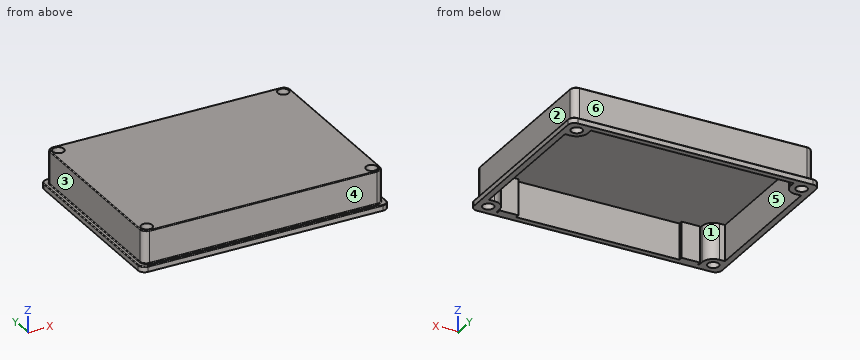
Autodesk Inventor part; units mm, degrees
ref_plane "YZ Plane" through (0, 0, 0) normal (1, 0, 0) x (0, 1, 0)
ref_plane "XZ Plane" through (0, 0, 0) normal (0, 1, 0) x (-1, 0, 0)
ref_plane "XY Plane" through (0, 0, 0) normal (0, 0, 1) x (1, 0, 0)
sketch "Sketch1" plane through (0, 0, 0) normal (0, 0, 1) x (1, 0, 0)
  line L0 (-150, 110) -> (150, 110)
  line L1 (150, 110) -> (150, -110)
  line L2 (150, -110) -> (-150, -110)
  line L3 (-150, -110) -> (-150, 110)
  line L4 (-150, 110) -> (150, -110) construction
  line L5 (150, 110) -> (-150, -110) construction
  point P0 (0, 0)
  dimension "d0" = 300
  dimension "d1" = 220
extrude "Extrusion1" add sketch "Sketch1" along normal blind 48
sketch "Sketch2" plane through (0, 0, 0) normal (0, 0, 1) x (1, 0, 0)
  line L0 (-155, -115) -> (155, -115)
  line L1 (155, -115) -> (155, 115)
  line L2 (155, 115) -> (-155, 115)
  line L3 (-155, 115) -> (-155, -115)
  line L4 (-155, -115) -> (155, 115) construction
  line L5 (155, -115) -> (-155, 115) construction
  point P0 (0, 0)
  dimension "d4" = 310
  dimension "d5" = 230
extrude "Extrusion2" add sketch "Sketch2" along normal blind 7
fillet "Fillet1" radius 8 8 edges at (-150, -110, 27.5) (-155, -115, 3.5) (155, -115, 3.5) (150, -110, 27.5) (155, 115, 3.5) (150, 110, 27.5) (-155, 115, 3.5) (-150, 110, 27.5)
fillet "Fillet2" radius 1 24 edges at (152.6569, -112.6569, 7) (155, 0, 7) (152.6569, 112.6569, 7) (0, 115, 7) (-152.6569, 112.6569, 7) (-155, 0, 7) (-152.6569, -112.6569, 7) (0, -115, 7) (147.6569, -107.6569, 7) (150, 0, 7) (147.6569, 107.6569, 7) (0, 110, 7) (-147.6569, 107.6569, 7) (-150, 0, 7) (-147.6569, -107.6569, 7) (0, -110, 7) (147.6569, -107.6569, 48) (150, 0, 48) (147.6569, 107.6569, 48) (0, 110, 48) (-147.6569, 107.6569, 48) (-150, 0, 48) (-147.6569, -107.6569, 48) (0, -110, 48)
sketch "Sketch3" plane through (0, 0, 0) normal (0, 0, 1) x (1, 0, 0)
  line L0 (-147.5, 107.5) -> (-126.5, 107.5) construction
  line L1 (147.5, 107.5) -> (147.5, 86.5) construction
  line L2 (147.5, -107.5) -> (126.5, -107.5) construction
  line L3 (-147.5, -107.5) -> (-147.5, -86.5) construction
  line L4 (-147.5, 107.5) -> (147.5, -107.5) construction
  line L5 (147.5, 107.5) -> (-147.5, -107.5) construction
  line L6 (-140.5, 100.5) -> (140.5, 100.5) construction
  line L7 (140.5, 100.5) -> (140.5, -100.5) construction
  line L8 (140.5, -100.5) -> (-140.5, -100.5) construction
  line L9 (-140.5, -100.5) -> (-140.5, 100.5) construction
  line L10 (-140.5, 100.5) -> (140.5, -100.5) construction
  line L11 (140.5, 100.5) -> (-140.5, -100.5) construction
  circle A0 centre (-140.5, -100.5) radius 14
  circle A1 centre (140.5, -100.5) radius 14
  circle A2 centre (140.5, 100.5) radius 14
  circle A3 centre (-140.5, 100.5) radius 14
  line L12 (-140.5, -86.5) -> (-147.5, -86.5)
  line L13 (-126.5, -100.5) -> (-126.5, -107.5)
  line L14 (126.5, -100.5) -> (126.5, -107.5)
  line L15 (140.5, -86.5) -> (147.5, -86.5)
  line L16 (-126.5, 100.5) -> (-126.5, 107.5)
  line L17 (-140.5, 86.5) -> (-147.5, 86.5)
  line L18 (126.5, 100.5) -> (126.5, 107.5)
  line L19 (140.5, 86.5) -> (147.5, 86.5)
  line L20 (-147.5, -86.5) -> (-147.5, 86.5)
  line L21 (-126.5, -107.5) -> (-147.5, -107.5) construction
  line L22 (126.5, -107.5) -> (-126.5, -107.5)
  line L23 (147.5, -86.5) -> (147.5, -107.5) construction
  line L24 (147.5, 86.5) -> (147.5, -86.5)
  line L25 (126.5, 107.5) -> (147.5, 107.5) construction
  line L26 (-126.5, 107.5) -> (126.5, 107.5)
  line L27 (-147.5, 86.5) -> (-147.5, 107.5) construction
  point P0 (0, 0)
  point P1 (0, 0)
  point P2 (0, 0)
  dimension "d10" = 295
  dimension "d11" = 215
  dimension "d16" = 281
  dimension "d17" = 201
  dimension "d18" = 28
extrude "Extrusion3" cut sketch "Sketch3" along normal blind 45 contours A0 L12 L20 L17 A3 L16 L26 L18 A2 L19 L24 L15 A1 L14 L22 L13
hole "Hole1" at (-140.5, -100.5, 0) direction (0, 0, 1) diameter 14 end through all
hole "Hole2" at (140.5, -100.5, 0) direction (0, 0, 1) diameter 14 end through all
hole "Hole3" at (-140.5, 100.5, 0) direction (0, 0, 1) diameter 14 end through all
hole "Hole4" at (140.5, 100.5, 0) direction (0, 0, 1) diameter 14 end through all
sketch "Sketch4" plane through (0, 0, 0) normal (0, 0, 1) x (1, 0, 0)
  line L0 (-125, -107.5) -> (-102, -107.5)
  line L1 (-102, -107.5) -> (-102, -102.5)
  line L2 (-102, -102.5) -> (-125, -102.5)
  line L3 (-125, -102.5) -> (-125, -107.5)
  line L4 (-126.5, -107.5) -> (126.5, -107.5)
  line L5 (0, -107.5) -> (0, 0) construction
  line L6 (125, -107.5) -> (102, -107.5)
  line L7 (102, -107.5) -> (102, -102.5)
  line L8 (102, -102.5) -> (125, -102.5)
  line L9 (125, -102.5) -> (125, -107.5)
  dimension "d57" = 23
  dimension "d58" = 5
  dimension "d59" = 204
extrude "Extrusion4" add sketch "Sketch4" along normal up to next
properties part number "caixa-gabinete-tampa" material "ABS Plastic"
Read the model definition and answer for the solid it produces. Units are mm, in the model's axes. Face numbers are marked on the shaded views. A direction names the side the tool comes from. Round coordinates to 2 decimals unless told otherwise and drop trailing zeros. Loops run counter-clockwise (first coordinate to the right, second up) from the corner with the lowest first, then second, coordinate; pieces in that order, holes last. Notation, with made-up numbers: (-34, 40) - (-13, 40) arc R30 ccw to (-13, 70) - close; hole circle Ø3 at (50, 1.25). An arc over 180 degrees is marked (long way). One line per question, with ' | ' between items. Start each with the question number.
Q1. Section B-B on y = -80 is taken. Give the vertices of the cut face in (x, z).
Q2. For a pull along X with two mould halves and no side action, classify the marked faces 1, 2 and 3 as +X half, -X half, draft (parallel to the pull), parting line (faces both ways), or undercut.
Q3. Section C-C on z = 37.5 is taken. Count the separate pieces of the cut face and the enclosed holes in it, plus the area to 3 significant figures.
Q4. Section A-A on x = 58.5 is taken. Give the vertices of the cut face in (y, z).
Q5. For the marked faces 4, 5 and 6, determine the directions among +Z, -Z, +X, -X, +Y, -Y from which every point of the face is accessible in a straight line to the end or side of a thin tool.
Q6. Find the intervals of material crossed by L1, parallel to Y at x = -140, z = 13; L2, parallel to X at y = -100, z = 36; L3, parallel to Y at x = 96.5, z = 25.5, in increasing order.
Q7. Flat-ended cylindrical pins translate along their axes: pin 1 (5.5 mm diameter, centred on y = -105.5, z = 15, fed in from -X); pin 2 (2 mm diameter, centred on x = -28.5, z = 32.5, fed in from -Y); pin 3 (1 mm diameter, centred on y = -85.5, z = 21.5, fed in from +X). Find the tip coordinate at first contact, or state that the pin passes through.
Established:
1) outline: (-155, 0) - (-147.5, 0) - (-147.5, 45) - (147.5, 45) - (147.5, 0) - (155, 0) - (155, 6) arc R1 ccw to (154, 7) - (151, 7) arc R1 cw to (150, 8) - (150, 47) arc R1 ccw to (149, 48) - (-149, 48) arc R1 ccw to (-150, 47) - (-150, 8) arc R1 cw to (-151, 7) - (-154, 7) arc R1 ccw to (-155, 6) - close
2) face 1: undercut | face 2: +X half | face 3: -X half
3) separate pieces: 1 | enclosed holes: 5 | area: 3,730 mm²
4) outline: (-115, 0) - (-107.5, 0) - (-107.5, 45) - (107.5, 45) - (107.5, 0) - (115, 0) - (115, 6) arc R1 ccw to (114, 7) - (111, 7) arc R1 cw to (110, 8) - (110, 47) arc R1 ccw to (109, 48) - (-109, 48) arc R1 ccw to (-110, 47) - (-110, 8) arc R1 cw to (-111, 7) - (-114, 7) arc R1 ccw to (-115, 6) - close
5) face 4: +Z, +X, -X, -Y | face 5: -Z | face 6: +Z, +X, -X, +Y
6) L1: -110 to -107.48, -93.52 to -86.51, 86.51 to 93.52, 107.48 to 110 | L2: -150 to -147.48, -133.52 to -126.51, 126.51 to 133.52, 147.48 to 150 | L3: -110 to -107.5, 107.5 to 110
7) pin 1: x = -149.96 | pin 2: y = -110 | pin 3: x = 150
